Autodesk Inventor part; units mm, degrees
ref_plane "YZ Plane" through (0, 0, 0) normal (1, 0, 0) x (0, 1, 0)
ref_plane "XZ Plane" through (0, 0, 0) normal (0, 1, 0) x (-1, 0, 0)
ref_plane "XY Plane" through (0, 0, 0) normal (0, 0, 1) x (1, 0, 0)
sketch "Sketch9" plane through (0, 0, 0) normal (0, 1, 0) x (-1, 0, 0)
  line L0 (25, 25) -> (-25, 25)
  line L1 (-25, 25) -> (-25, -25)
  line L2 (-25, -25) -> (25, -25)
  line L3 (25, -25) -> (25, 25)
  line L4 (25, 25) -> (-25, -25) construction
  line L5 (-25, 25) -> (25, -25) construction
  line L6 (-23, 23) -> (23, 23)
  line L7 (23, 23) -> (23, -23)
  line L8 (23, -23) -> (-23, -23)
  line L9 (-23, -23) -> (-23, 23)
  point P0 (0, 0)
  dimension "d172" = 50
  dimension "d173" = 50
  dimension "d174" = 2
extrude "Extrusion3" add sketch "Sketch9" against normal blind 805
sketch "Sketch10" plane through (0, 0, 0) normal (1, 0, 0) x (0, 1, 0)
  line L0 (0, 25) -> (0, -25) construction
  line L1 (0, 25) -> (-805, 25) construction
  line L2 (-805, -25) -> (-805, 25) construction
  line L3 (0, -25) -> (-805, -25) construction
  line L4 (-800, 8.5) -> (-783, 8.5)
  line L5 (-783, 8.5) -> (-783, -8.5)
  line L6 (-783, -8.5) -> (-800, -8.5)
  line L7 (-800, -8.5) -> (-800, 8.5)
  line L8 (-800, 8.5) -> (-783, -8.5) construction
  line L9 (-783, 8.5) -> (-800, -8.5) construction
  circle A0 centre (-791.5, 0) radius 8.5
  line L10 (0, 25) -> (0, -25)
  point P0 (0, 0)
  point P1 (0, 0)
  point P2 (-805, 0)
  dimension "d177" = 17
  dimension "d178" = 17
  dimension "d191" = 5
extrude "Extrusion4" cut sketch "Sketch10" along normal through all contours A0
pattern_linear "Rectangular Pattern4" count 7 spacing 125 along (0, 1, 0) of "Extrusion4"
properties part number "TKS 3536 FDS WAY tube6" material "Stainless Steel"
Could you check a few things on this model? Use its own coordinates, in mm. A direction names the side the tool comes from. Give positions to 0.01 mm unless a question says otherwise; leave off trailing zeros. Order: outer loops, then holes, each group sorted by start corner. A loop starts at its lowest first (then second) coordinate and runs counter-clockwise, first axis right, second up. Notation, with made-up numbers: (-13.75, 72) - (9.25, 72) arc R22 ccw to (9.25, 97) - close; hole circle Ø7 at (65.5, 17.25). An arc over 180 degrees is marked (long way). One line per question, with ' | ' between items. Start each with the question number.
Item 1: I need wall thicknesses on probe 1 along Z at (x, y) = (24.25, -416.5); probe 2 along X at (y, z) = (-679, -10). Which ranges of each line are inside material? Lowest first, please. Write a range as [from, to].
Item 2: I want a section at D-D on y = -666.5. Write out the boundary of the cut face in (x, z).
Item 3: I'm going to push a flat-ended pin straight in: pin 1 Ø10 at (x, z) = (16, -17.5) entering from +Y. Where does the tip first touch, or does it pass through?
Item 4: I want a section at B-B on z = 15. Write out the boundary of the cut face in (x, y).
Item 5: Thinking about a two-plate mould opening in X: for faces 4 (the flat face through (2, -805, -24)), 5 (the flat face through (-25, -397, 0)), 6 (the flat face through (-23, -397, 0)), which applies, pulls with the +X half, pulls with the -X half, needs draft (parallel to the pull), parting line crosses it, or undercut?
Item 6: I want a section at A-A on y = -206.5. Write out the boundary of the cut face in (x, z), then the cut area to 3 significant figures.
Item 7: For faces 1 (the cylindrical face through (24, -550, 0)), 2 (the flat face through (25, -397, 0)), 3 (the flat face through (0, -397, 23)), which set-ups out of +Z, -Z, +X, -X, +Y, -Y let a thin tool reach every point of the face, with its end or its side?
Item 8: I want a section at C-C on x = 14. Write out the boundary of the cut face in (y, z), then the cut area to 3 significant figures.
Verdict:
1) probe 1: [-25, -8.5], [8.5, 25] | probe 2: [-25, -23], [23, 25]
2) outline: (-25, -25) - (25, -25) - (25, -8.5) - (23, -8.5) - (23, -23) - (-23, -23) - (-23, 23) - (23, 23) - (23, 8.5) - (25, 8.5) - (25, 25) - (-25, 25) - close
3) pin 1: through
4) outline: (-25, -805) - (-23, -805) - (-23, 0) - (-25, 0) - close; (23, -805) - (25, -805) - (25, 0) - (23, 0) - close
5) face 4: needs draft | face 5: pulls with the -X half | face 6: undercut
6) outline: (-25, -25) - (25, -25) - (25, 25) - (-25, 25) - close; hole (-23, -23) - (23, -23) - (23, 23) - (-23, 23) - close | area: 384 mm^2
7) face 1: +X | face 2: +Z, -Z, +X, +Y, -Y | face 3: +Y, -Y
8) outline: (-805, -25) - (0, -25) - (0, -23) - (-805, -23) - close; (-805, 23) - (0, 23) - (0, 25) - (-805, 25) - close | area: 3,220 mm^2
